from build123d import *

# Parameters (mm, degrees)
SKETCH_R        = 1.75
SKETCH_R_2      = 1.125
PAD_DEPTH       = 4
CHAMFER_SIZE    = 1
CHAMFER001_SIZE = 0.5
FILLET_R        = 2


with BuildPart() as part:
    # Sketch → Pad (new body)
    with BuildSketch(Plane.XY):
        Polygon((0, 0), (19, 0), (19, 19), (0, 19), (-20, 19), (-20, 8), (0, 8), align=None)
        with Locations((5, 3)):
            Circle(SKETCH_R, mode=Mode.SUBTRACT)
        with Locations((6, 13.6)):
            Circle(SKETCH_R, mode=Mode.SUBTRACT)
        with Locations((-2.9, 17)):
            Circle(SKETCH_R_2, mode=Mode.SUBTRACT)
        with Locations((-17.1, 17)):
            Circle(SKETCH_R_2, mode=Mode.SUBTRACT)
    extrude(amount=PAD_DEPTH)

    # Chamfer
    chamfer_edges = [part.edges().sort_by_distance(p)[0] for p in [
        (4.25, 13.6, 4),
        (3.25, 3, 4),
    ]]
    chamfer(chamfer_edges, length=CHAMFER_SIZE)

    # Chamfer001
    chamfer001_edges = [part.edges().sort_by_distance(p)[0] for p in [
        (-4.025, 17, 4),
        (-18.225, 17, 4),
    ]]
    chamfer(chamfer001_edges, length=CHAMFER001_SIZE)

    # Fillet
    fillet_edges = [part.edges().sort_by_distance(p)[0] for p in [
        (0, 0, 2),
        (-20, 8, 2),
        (-20, 19, 2),
    ]]
    fillet(fillet_edges, radius=FILLET_R)


solid = part.part
Work out the finished part from the listing and answer in its coordinate system (mm). A direction names the side the tool comes from. Coordinates: 2 decimals unless noted, no trailing zeros. Write each loop counter-clockwise with the first axis right and the second up, starting at its lowest first coordinate (ties: lowest second). Pieces come first, ordered by that corner, then holes. Notation, with made-up numbers: M 36.5,-33.75 L 81.5,-33.75 A26 cw 81.5,-6.75 Z; hole C -38,-27.75 d2. An arc over 180 degrees is marked long. Use one line per item in the form item = value. Start each with the question number.
1. The part is cut by section D-D (x = -8.5). Give the vertices of the cut face in (y, z), plus the area to 3 significant figures.
2. Straight lines are drawn through the part: probe 1 along Y at (x, z) = (6, 2.15); probe 2 along Y at (x, z) = (5, 2.3); probe 3 along Y at (x, z) = (-17.1, 0.7) (3 decimals). For each, find the intervals that lie inside material, in ascending order. Write a range as from..to.
3. The part is cut by section C-C (z = 1.2). Give the vertices of the cut face in (x, y) (3 decimals), plus the area to 3 significant figures.
4. The part is cut by section B-B (y = 3). Give the vertices of the cut face in (x, z).
5. The mould has two halves that part along X. Classify faces 1 (the face through (3.61, 1.94, 1.48)), 2 (the face through (1, 19, 2)), 3 (the face through (5.62, 11.89, 1.48)), 4 (the face through (-19.4, 8.57, 2.03)): released by +X, released by -X, zero draft, split by the parting line, or undercut.
6. The part is cut by section A-A (x = -17.1). Give the vertices of the cut face in (y, z) (3 decimals).
7. A tool of negligible diameter and unlimited length cuts with its end or side. For faces 5 (the face through (19, 9, 2)), 6 (the face through (0, 5, 2)), from which of +Z, -Z, +X, -X, +Y, -Y can it reach the whole face along a straight path? Write none if from no direction.
Evaluation:
q1.outline = M 8,0 L 19,0 L 19,4 L 8,4 Z
q1.area = 44.0 mm^2
q2.probe_1 = 0..1.56, 4.44..11.85, 15.35..19
q2.probe_2 = 0..1.25, 4.75..12.16, 15.04..19
q2.probe_3 = 8..15.875, 18.125..19
q3.outline = M -20,10 A2 ccw -18,8 L 0,8 L 0,2 A2 ccw 2,0 L 19,0 L 19,19 L -18,19 A2 ccw -20,17 Z; hole C -17.1,17 d2.25; hole C -2.9,17 d2.25; hole C 5,3 d3.5; hole C 6,13.6 d3.5
q3.area = 551 mm^2
q4.outline = M 0,0 L 3.25,0 L 3.25,3 L 2.25,4 L 0,4 Z; M 6.75,0 L 19,0 L 19,4 L 7.75,4 L 6.75,3 Z
q5.face_1 = undercut
q5.face_2 = zero draft
q5.face_3 = undercut
q5.face_4 = released by -X
q6.outline = M 8,0 L 15.875,0 L 15.875,3.5 L 15.375,4 L 8,4 Z; M 18.125,0 L 19,0 L 19,4 L 18.625,4 L 18.125,3.5 Z
q7.face_5 = +Z, -Z, +X, +Y, -Y
q7.face_6 = +Z, -Z, -X, -Y
